Build history of the part. All positions in model axes, mm. A direction names the side the tool comes from. Round coordinates to 2 decimals unless told otherwise and drop trailing zeros. Write each loop counter-clockwise with the first axis right and the second up, starting at its lowest first coordinate (ties: lowest second). Pieces come first, ordered by that corner, then holes. Notation, with made-up numbers: M 29,26 L 74,26 A17 cw 74,52 Z; hole C -34,-10.75 d2. An arc over 180 degrees is marked long. Write item = value, one per line. Start each with the question number.
Q1. Pull direction X, two halves, no side cores. Call faces 1 (the flat face through (-4, 1, 12.5)), 2 (the cylindrical face through (11.99, 1.48, 9.65)), 3 (the flat face through (-10.5, 1, 0)): released by +X, released by -X, zero draft, split by the parting line, or undercut.
Q2. Probe L1, parallel to X at y = 2.2, z = 0; L2, parallel to X at y = 2.7, z = 1.5; L3, parallel to X at y = 0.45, z = 2.25. List the from-to ranges inside material, lowest first.
Q3. Tool access for faces 4 (the flat face through (-7.5, 1, 0)), 5 (the cylindrical face through (-14, 1, 12)): list every direction of +Z, -Z, +X, -X, +Y, -Y with a clear straight run to the whole face (end or side of a thin tool).
Q4. Drop a flat-ended pin along its axis: P1, Ø4, axis at x = 5, z = 0, coming from the +Y side. Give the stop position or say it passes through.
Q5. Band-saw the part on C-C on z = -3.25. Write the cut outline in (x, y).
Q6. Band-saw the part on A-A on y = 0.55. Write the cut outline in (x, z), plus the area to 3 significant figures.
Q7. Band-saw the part on B-B on z = 0. Write the cut outline in (x, y), plus the area to 3 significant figures.
Q8. Band-saw the part on D-D on x = 9. Write the cut outline in (y, z).
```python
from build123d import *

# Parameters (mm, degrees)
SKETCH1_R           = 1.75
SKETCH1_W           = 3
SKETCH1_H           = 10
BOSS_EXTRUDE1_DEPTH = 3


with BuildPart() as part:
    # Sketch1 → Boss-Extrude1 (new body)
    with BuildSketch(Plane(origin=(0, 0, 0), x_dir=(1, 0, 0), z_dir=(0, 1, 0))):
        with BuildLine():
            Line((-12.5, -12.5), (5, -12.5))
            ThreePointArc((5, -12.5), (12.071067812, -9.571067812), (15, -2.5))
            Line((15, -2.5), (15, 2.5))
            ThreePointArc((15, 2.5), (12.071067812, 9.571067812), (5, 12.5))
            Line((5, 12.5), (-12.5, 12.5))
            ThreePointArc((-12.5, 12.5), (-14.267766953, 11.767766953), (-15, 10))
            Line((-15, 10), (-15, -10))
            ThreePointArc((-15, -10), (-14.267766953, -11.767766953), (-12.5, -12.5))
        make_face()
        with Locations(Location((5, 0, 0), (0, 0, 270))):
            Circle(SKETCH1_R, mode=Mode.SUBTRACT)
        with Locations((-9, 0)):
            Rectangle(SKETCH1_W, SKETCH1_H, mode=Mode.SUBTRACT)
    extrude(amount=BOSS_EXTRUDE1_DEPTH)


solid = part.part
```
Conclusion:
q1.face_1 = zero draft
q1.face_2 = released by +X
q1.face_3 = undercut
q2.L1 = -15 to -10.5, -7.5 to 3.25, 6.75 to 15
q2.L2 = -15 to -10.5, -7.5 to 4.1, 5.9 to 15
q2.L3 = -15 to -10.5, -7.5 to 15
q3.face_4 = +Y, -Y
q3.face_5 = +Z, -X, +Y, -Y
q4.P1 = 3
q5.outline = M -15,0 L -10.5,0 L -10.5,3 L -15,3 Z; M -7.5,0 L 14.97,0 L 14.97,3 L -7.5,3 Z
q6.outline = M -15,-10 A2.5 ccw -12.5,-12.5 L 5,-12.5 A10 ccw 15,-2.5 L 15,2.5 A10 ccw 5,12.5 L -12.5,12.5 A2.5 ccw -15,10 Z; hole M -10.5,-5 L -7.5,-5 L -7.5,5 L -10.5,5 Z; hole C 5,0 d3.5
q6.area = 665 mm^2
q7.outline = M -15,0 L -10.5,0 L -10.5,3 L -15,3 Z; M -7.5,0 L 3.25,0 L 3.25,3 L -7.5,3 Z; M 6.75,0 L 15,0 L 15,3 L 6.75,3 Z
q7.area = 70.5 mm^2
q8.outline = M 0,-11.67 L 3,-11.67 L 3,11.67 L 0,11.67 Z
